from build123d import *

# Parameters (mm, degrees)
TAPPED_HOLE1_REACH  = 103.897
TAPPED_HOLE1_BORE_R = 2.1
CIRPATTERN1_COUNT   = 2
CIRPATTERN1_ANGLE   = 90
DIAMETER_HOLE1_D    = 5.5
DIAMETER_HOLE2_D    = 5.5


with BuildPart() as part:
    # Sketch1 → Revolve1 (revolve)
    with BuildSketch(Plane.XY, mode=Mode.PRIVATE) as revolve1_sk:
        Polygon((0, 12.5), (0, 27.5), (8, 27.5), (8, 16.5), (38, 16.5), (38, 12.5), align=None)
    revolve(revolve1_sk.sketch.rotate(Axis((0, 0, 0), (1, 0, 0)), 90), axis=Axis((0, 0, 0), (1, 0, 0)))

    # Tapped Hole1 bore → Tapped Hole1 (cut, up to next)
    with BuildSketch(Plane(origin=(84.688297546, 3.217458949, 20.11706483), x_dir=(1, 0, 0), z_dir=(0, 0.7071067811865488, 0.7071067811865464)), mode=Mode.PRIVATE) as tapped_hole1_sk1:
        with Locations((-61.688297546, 11.949825918)):
            Circle(TAPPED_HOLE1_BORE_R)
    tapped_hole1_tool1 = extrude(tapped_hole1_sk1.sketch, amount=-TAPPED_HOLE1_REACH, mode=Mode.PRIVATE) & part.part
    tapped_hole1 = tapped_hole1_tool1.solids().sort_by_distance((23, 11.667262, 11.667262))[0]
    add(tapped_hole1, mode=Mode.SUBTRACT)

    # CirPattern1: Tapped Hole1 ×2 about axis
    cirpattern1_axis = Axis((0, 0, 0), (1, 0, 0))
    for i in range(1, CIRPATTERN1_COUNT):
        add(tapped_hole1.rotate(cirpattern1_axis, i * CIRPATTERN1_ANGLE / (CIRPATTERN1_COUNT - 1)), mode=Mode.SUBTRACT)

    # Diameter Hole1 (through all)
    with Locations(Plane(origin=(8, 0, 0), x_dir=(0, 0, -1), z_dir=(1, 0, 0))):
        with Locations((0, 22), (0, -22)):
            Hole(DIAMETER_HOLE1_D / 2)

    # Diameter Hole2 (through all)
    with Locations(Plane(origin=(8, 0, 0), x_dir=(0, 0, -1), z_dir=(1, 0, 0))):
        with Locations((-22, 0), (22, 0)):
            Hole(DIAMETER_HOLE2_D / 2)


solid = part.part
Read the model definition and answer for the solid it produces. Units are mm, in the model's axes. A direction names the side the tool comes from. Coordinates: 2 decimals unless noted, no trailing zeros. Order: outer loops, then holes, each group sorted by start corner. A loop starts at its lowest first (then second) coordinate and runs counter-clockwise, first axis right, second up. Notation, with made-up numbers: M -32.75,40.25 L 19.25,40.25 A11 cw 19.25,52.25 Z; hole C 83.25,-17 d1. An arc over 180 degrees is marked long. Put each result on its own line as item: value. Start each with the question number.
Item 1: For faces 1 (the face through (23.21, -4.956, 15.738)), 2 (the face through (3.944, -19.273, -0.358)), determine the directions among +Z, -Z, +X, -X, +Y, -Y from which every point of the face is accessible in a straight line to the end or side of a thin tool.
Item 2: Given pin 1 Ø5 at (y, z) = (-19, 20) entering from +X; pin 2 Ø1 at (x, z) = (21.5, 8) entering from -Y; pin 3 Ø4 at (x, z) = (16.5, -15) entering from -Y, each flat-ended and moving along its own axis, determine where each tip first touches the part or whether it passes through.
Item 3: The mould has two halves that part along Y. Classify faces 3 (the face through (20.902, 10.276, 10.146)), 4 (the face through (4.056, 24.397, 12.69)), 5 (the face through (38, -3.7, -12.3)): +Y half, -Y half, draft (parallel to the pull), parting line (faces both ways), or undercut.
Item 4: Section A-A, the plane y = 0 is taken. Determine the outline of the cut face in (x, z).
Item 5: Consider probe 1 along Y at (x, z) = (3.75, 0); probe 2 along Y at (x, z) = (5.5, 22); probe 3 along X at (y, z) = (15, -16). Determine where each line is inside the solid, lowest interval first. Write a range as [from, to].
Item 6: Section B-B, the plane z = -22 is taken. Determine the outline of the cut face in (x, y).
Computed:
1. face 1: +X
1. face 2: +X, -X
2. pin 1: stops at x = 8
2. pin 2: stops at y = -14.7
2. pin 3: stops at y = -10.16
3. face 3: undercut
3. face 4: parting line
3. face 5: draft
4. outline: M 0,-27.5 L 8,-27.5 L 8,-24.75 L 0,-24.75 Z; M 0,-19.25 L 8,-19.25 L 8,-16.5 L 38,-16.5 L 38,-12.5 L 0,-12.5 Z; M 0,12.5 L 38,12.5 L 38,16.5 L 8,16.5 L 8,19.25 L 0,19.25 Z; M 0,24.75 L 8,24.75 L 8,27.5 L 0,27.5 Z
5. probe 1: y = [-27.5, -24.75], [-19.25, -12.5], [12.5, 19.25], [24.75, 27.5]
5. probe 2: y = [-16.5, -2.75], [2.75, 16.5]
5. probe 3: x = [0, 8]
6. outline: M 0,-16.5 L 8,-16.5 L 8,-2.75 L 0,-2.75 Z; M 0,2.75 L 8,2.75 L 8,16.5 L 0,16.5 Z
